from build123d import *
from build123d.topology import SkipClean

# Parameters (mm, degrees)
CUT_EXTRUDE1_DEPTH      = 26.980762114
CUT_EXTRUDE1_DEPTH_BACK = 26.980762114
SKETCH2_R               = 2.25
CUT_EXTRUDE2_DEPTH      = 26.88315089
CUT_EXTRUDE3_DEPTH      = 31.577337854
CIRPATTERN1_COUNT       = 6
CHAMFER1_SIZE           = 4


with BuildPart() as part:
    # Sketch1 → Revolve1 (revolve)
    with BuildSketch(Plane(origin=(0, 0, 0), x_dir=(1, 0, 0), z_dir=(0, 1, 0))):
        with BuildLine():
            Line((0, 15), (0, 13))
            ThreePointArc((0, 13), (9.192388155, 9.192388155), (13, 0))
            Line((13, 0), (15, 0))
            ThreePointArc((15, 0), (10.606601718, 10.606601718), (0, 15))
        make_face()
    revolve(axis=Axis((0, 0, -15), (0, 0, 1)))

    # Sketch2 → Cut-Extrude1 (cut, two sides: drawn at the far end of the back side and taken through both)
    with BuildSketch(Plane.XY.offset(-CUT_EXTRUDE1_DEPTH_BACK)):
        Circle(SKETCH2_R)
    extrude(amount=CUT_EXTRUDE1_DEPTH + CUT_EXTRUDE1_DEPTH_BACK, mode=Mode.SUBTRACT)

    # Sketch3 → Cut-Extrude2 (cut, symmetric)
    with BuildSketch(Plane(origin=(0, 0, 0), x_dir=(1, 0, 0), z_dir=(0, 1, 0))):
        Polygon((-2.5, -55.877554425), (-2.5, 0), (-2.5, 12), (2.5, 12), (2.5, 0), (2.5, -55.877554425), (2.5, -167.632663274), (-2.5, -167.632663274), align=None)
    cut_extrude2 = extrude(amount=CUT_EXTRUDE2_DEPTH, both=True, mode=Mode.SUBTRACT)

    # Sketch5 → Cut-Extrude3 (cut, symmetric)
    with BuildSketch(Plane(origin=(0, 9, -12), x_dir=(-1, 0, 0), z_dir=(0, 0.6000000000000006, -0.7999999999999996))):
        with BuildLine():
            Line((-2.5, 0), (2.5, 0))
            ThreePointArc((2.5, 0), (0, -2.5), (-2.5, 0))
        make_face()
    cut_extrude3 = extrude(amount=CUT_EXTRUDE3_DEPTH, both=True, mode=Mode.SUBTRACT)

    # CirPattern1: Cut-Extrude2, Cut-Extrude3 ×6 about axis
    with SkipClean():  # the faces are left unmerged after this step: merging them gives an invalid solid
        cirpattern1_axis = Axis((0, 0, -15), (0, 0, 1))
        add([cut_extrude2.rotate(cirpattern1_axis, i * 360 / CIRPATTERN1_COUNT) for i in range(1, CIRPATTERN1_COUNT)], mode=Mode.SUBTRACT)
        add([cut_extrude3.rotate(cirpattern1_axis, i * 360 / CIRPATTERN1_COUNT) for i in range(1, CIRPATTERN1_COUNT)], mode=Mode.SUBTRACT)

    # Chamfer1
    chamfer1_edges = [part.edges().sort_by_distance(p)[0] for p in [
        (-2.5, -13.77377514, 0),
        (-2.5, 13.77377514, 0),
        (2.5, -13.77377514, 0),
        (2.5, 13.77377514, 0),
        (-13.178439177, 4.721824061, 0),
        (10.678439177, -9.051951079, 0),
        (13.178439177, -4.721824061, 0),
        (-10.678439177, 9.051951079, 0),
        (-10.678439177, -9.051951079, 0),
        (13.178439177, 4.721824061, 0),
        (10.678439177, 9.051951079, 0),
        (-13.178439177, -4.721824061, 0),
    ]]
    chamfer(chamfer1_edges, length=CHAMFER1_SIZE - 0.0001)  # a hair under: the kernel refuses the full size


solid = part.part
Geometry: final body of the model. Coordinates: model frame, mm. A direction names the side the tool comes from. Give positions to 0.01 mm unless a question says otherwise; leave off trailing zeros. Loops run counter-clockwise (first coordinate to the right, second up) from the corner with the lowest first, then second, coordinate; pieces in that order, holes last. Notation, with made-up numbers: (40, 62) - (52, 62) arc R24 ccw to (52, 73) - close; hole circle Ø3 at (68, 59). An arc over 180 degrees is marked (long way). One line per question, with ' | ' between items. Start each with the question number.
(1) Section query D-D on y = -0.5. Return loops of the section in (x, z), then the cut area to 3 significant figures.
(2) Section query A-A on y = -9.75. Return loops of the section in (x, z).
(3) Section query B-B on z = -3. Return loops of the section in (x, y), then the cut area to 3 significant figures.
(4) Ray query, line 1 (Y direction, x = 7.75, z = -3.25); line 2 (X direction, y = 2.25, z = -6.75); line 3 (X direction, y = 0, z = -13.65). Return the intervals inside material, ascending. Write a range as from..to.
(5) Reachability of faces 4 (the flat face through (-7.45, 7.19, -8.28)), 5 (the flat face through (-13.57, 2.67, -2.03)), 6 (the flat face through (-4.8, 2.7, -12)), 7 (the flat face through (-2.5, -10.4, -8.3)), 8 (the flat face through (13.57, -2.67, -2.03)) from +Z, -Z, +X, -X, +Y, -Y: full face, straight path, thin tool, end or side. Return the list, or none.
(6) Pull-direction query (Y, two-part tool) for faces 1 (the cylindrical face through (5.65, -3.2, -12.82)), 2 (the flat face through (-13.63, -2.64, -1.97)), 3 (the flat face through (13.63, 2.64, -1.97)); classes: released by +Y, released by -Y, zero draft, split by the parting line, or undercut.
(7) Contact query for flat-ended pins moving along their axis: pin 1 (1.5 mm diameter, centred on y = 8.5, z = -2.5, fed in from +X); pin 2 (2 mm diameter, centred on x = 1, y = 6.5, fed in from +Z); pin 3 (1 mm diameter, centred on x = 6.5, y = -6.5, fed in from -Z); pin 4 (2.5 mm diameter, centred on y = -10.5, z = -8, fed in from +X). Output: stop coordinate, or through.
(8) Section query C-C on x = 0. Return loops of the section in (y, z) (3 decimals), then the cut area to 3 significant figures.
The answers:
1) outline: (-14.99, 0) arc R14.99 ccw to (-2.19, -14.83) - (-2.19, -12.8) arc R12.99 cw to (-4.97, -12) - (-5.87, -12) - (-5.87, -11.59) arc R12.99 cw to (-12.98, -0.44) - (-13.87, 0) - close; (2.19, -14.83) arc R14.99 ccw to (14.99, 0) - (13.87, 0) - (12.98, -0.44) arc R12.99 cw to (5.87, -11.59) - (5.87, -12) - (4.97, -12) arc R12.99 cw to (2.19, -12.8) - close | area: 78.4 mm2
2) outline: (-10.85, -3.48) arc R11.4 ccw to (-2.5, -11.12) - (-2.5, -8.23) arc R8.6 cw to (-8.31, -2.21) - close; (2.5, -11.12) arc R11.4 ccw to (10.85, -3.48) - (8.31, -2.21) arc R8.6 cw to (2.5, -8.23) - close
3) outline: (-14.11, -4.11) - (-12.28, -3.05) arc R12.65 cw to (-12.28, 3.05) - (-14.11, 4.11) arc R14.7 ccw to start; (-10.61, -10.17) arc R14.7 ccw to (-3.5, -14.27) - (-3.5, -12.16) arc R12.65 cw to (-8.78, -9.11) - close; (-10.61, 10.17) - (-8.78, 9.11) arc R12.65 cw to (-3.5, 12.16) - (-3.5, 14.27) arc R14.7 ccw to start; (3.5, -14.27) arc R14.7 ccw to (10.61, -10.17) - (8.78, -9.11) arc R12.65 cw to (3.5, -12.16) - close; (3.5, 12.16) arc R12.65 cw to (8.78, 9.11) - (10.61, 10.17) arc R14.7 ccw to (3.5, 14.27) - close; (12.28, -3.05) - (14.11, -4.11) arc R14.7 ccw to (14.11, 4.11) - (12.28, 3.05) arc R12.65 cw to start | area: 88.9 mm2
4) line 1: -12.42..-9.92, 9.92..12.42 | line 2: -13.21..-10.88, 10.88..13.21 | line 3: -6.22..-2.25, 2.25..6.22
5) face 4: +Z, -X | face 5: +Z, +Y | face 6: +Z | face 7: +Z, +Y, -Y | face 8: +Z, -Y
6) face 1: undercut | face 2: released by -Y | face 3: released by +Y
7) pin 1: through | pin 2: z = -12 | pin 3: z = -12.2 | pin 4: x = 9.07
8) outline: (-6.874, -13.332) arc R15 ccw to (-2.25, -14.83) - (-2.25, -12.804) arc R13 cw to (-5, -12) - (-5.875, -12) - close; (2.25, -14.83) arc R15 ccw to (6.874, -13.332) - (5.875, -12) - (5, -12) arc R13 cw to (2.25, -12.804) - close | area: 16.7 mm2
